Can you work these out from the model? Positions are in its coordinate system, mm. A direction names the side the tool comes from. Coordinates: 2 decimals unless noted, no trailing zeros. Loops run counter-clockwise (first coordinate to the right, second up) from the corner with the lowest first, then second, coordinate; pieces in that order, holes last. Notation, with made-up numbers: M 25,79.25 L 62,79.25 A32 cw 62,112.25 Z; hole C 59,53 d8. An arc over 180 degrees is marked long. Answer as a JSON object with one key per item and string values. Group by question number.
Item 1: Suppose I cut it at B-B (y = 0). Write out the boundary of the cut face in (x, z).
Item 2: Suppose I cut it at C-C (y = -9). Write out the boundary of the cut face in (x, z).
Item 3: If I drill on line 1 (X direction, y = 15.5, z = 1.9); line 2 (X direction, y = 15.5, z = 6.45), over which ranges is the centre line in solid material (lowest first)?
Item 4: I'm going to push flat-ended pins straight in: pin 1 Ø1.1 at (x, z) = (22, 2) entering from -Y; pin 2 Ø1 at (y, z) = (-6.5, 7) entering from +X; pin 3 Ø4 at (x, y) = (-14.5, 15.5) entering from -Z; pin 4 Ø1.8 at (x, z) = (24.5, 1.5) entering from +Y. Where does each tip first touch, or does it pass through?
Item 5: We'd pull the mould along Y, two halves only. Please class faces 1 (the cylindrical face through (-14, 15.43, 7.33)), 2 (the cylindrical face through (20.994, 16.097, 4.867)), 3 (the flat face through (18.7, -18.6, 4.7)), 4 (the flat face through (19, 8.2, 7)): +Y half, -Y half, draft (parallel to the pull), parting line (faces both ways), or undercut.
Item 6: Suppose I cut it at A-A (z = 8). Write out the boundary of the cut face in (x, y).
Item 7: Which directions (+Z, -Z, +X, -X, +Y, -Y) give clear straight access to the entire face, cutting with the end or side of a thin tool? Please do faces 5 (the cylindrical face through (17, -15.57, 7.33)), 6 (the flat face through (19, -8.2, 7)), 7 (the flat face through (-14, 17, 5)), 8 (the flat face through (21.15, 12, 5)).
```python
from build123d import *

# Parameters (mm, degrees)
SKETCH116_W      = 42.3
SKETCH116_H      = 42.3
PAD048_DEPTH     = 9.6
SKETCH118_W      = 4.3
SKETCH118_H      = 16.4
PAD001_DEPTH     = 3.6
CHAMFER005_SIZE  = 5
FILLET_R         = 2
HOLE_D           = 3
HOLE_DEPTH       = 25
HOLE_CBORE_D     = 5
HOLE_CBORE_DEPTH = 5
SKETCH013_W      = 16.4
SKETCH013_H      = 6
POCKET013_DEPTH  = 4


with BuildPart() as part:
    # Sketch116 → Pad048 (new body)
    with BuildSketch(Plane.XY):
        Rectangle(SKETCH116_W, SKETCH116_H)
    extrude(amount=PAD048_DEPTH)

    # Sketch118 → Pad001 (join)
    with BuildSketch(Plane.XY):
        with Locations((23.3, 0)):
            Rectangle(SKETCH118_W, SKETCH118_H)
    extrude(amount=PAD001_DEPTH)

    # Chamfer005
    chamfer005_edges = [part.edges().sort_by_distance(p)[0] for p in [
        (21.15, -21.15, 4.8),
        (-21.15, -21.15, 4.8),
        (-21.15, 21.15, 4.8),
        (21.15, 21.15, 4.8),
    ]]
    chamfer(chamfer005_edges, length=CHAMFER005_SIZE)

    # Fillet
    fillet_edges = [part.edges().sort_by_distance(p)[0] for p in [
        (16.15, -21.15, 4.8),
        (21.15, -16.15, 4.8),
        (21.15, 16.15, 4.8),
        (16.15, 21.15, 4.8),
        (-16.15, 21.15, 4.8),
        (-21.15, 16.15, 4.8),
        (-16.15, -21.15, 4.8),
        (-21.15, -16.15, 4.8),
    ]]
    fillet(fillet_edges, radius=FILLET_R)

    # Hole
    with Locations(Plane(origin=(0, 0, 0), x_dir=(1, 0, 0), z_dir=(0, 0, -1))):
        with Locations((-15.5, 15.5), (15.5, 15.5), (15.5, -15.5), (-15.5, -15.5)):
            CounterBoreHole(HOLE_D / 2, HOLE_CBORE_D / 2, HOLE_CBORE_DEPTH, depth=HOLE_DEPTH)

    # Sketch013 (on Face11 of Hole) → Pocket013 (cut)
    with BuildSketch(Plane.YZ.offset(21.15)):
        with Locations((0, 6.6)):
            Rectangle(SKETCH013_W, SKETCH013_H)
    extrude(amount=-POCKET013_DEPTH, mode=Mode.SUBTRACT)


solid = part.part
```
From the geometry:
{
 "1": {"outline": "M -21.15,0 L 25.45,0 L 25.45,3.6 L 17.15,3.6 L 17.15,9.6 L -21.15,9.6 Z"},
 "2": {"outline": "M -21.15,0 L 21.15,0 L 21.15,9.6 L -21.15,9.6 Z"},
 "3": {"line 1": "-21.14 to -18, -13 to 13, 18 to 21.14", "line 2": "-21.14 to -17, -14 to 14, 17 to 21.14"},
 "4": {"pin 1": "y = -8.2", "pin 2": "x = 17.15", "pin 3": "z = 0", "pin 4": "y = 8.2"},
 "5": {"face 1": "undercut", "face 2": "+Y half", "face 3": "-Y half", "face 4": "undercut"},
 "6": {"outline": "M -21.15,-15.32 A2 ccw -20.56,-16.74 L -16.74,-20.56 A2 ccw -15.32,-21.15 L 15.32,-21.15 A2 ccw 16.74,-20.56 L 20.56,-16.74 A2 ccw 21.15,-15.32 L 21.15,-8.2 L 17.15,-8.2 L 17.15,8.2 L 21.15,8.2 L 21.15,15.32 A2 ccw 20.56,16.74 L 16.74,20.56 A2 ccw 15.32,21.15 L -15.32,21.15 A2 ccw -16.74,20.56 L -20.56,16.74 A2 ccw -21.15,15.32 Z; hole C -15.5,-15.5 d3; hole C -15.5,15.5 d3; hole C 15.5,-15.5 d3; hole C 15.5,15.5 d3"},
 "7": {"face 5": "+Z, -Z", "face 6": "+Z, +X", "face 7": "-Z", "face 8": "+Z, -Z, +X, +Y"}
}
